Part model, mm, in its own coordinate system. A direction names the side the tool comes from. Give positions to 0.01 mm unless a question says otherwise; leave off trailing zeros. Write each loop counter-clockwise with the first axis right and the second up, starting at its lowest first coordinate (ties: lowest second). Pieces come first, ordered by that corner, then holes. Notation, with made-up numbers: M 20,-8.75 L 62,-8.75 A23 cw 62,20.25 Z; hole C -29.5,64.5 d1. An arc over 180 degrees is marked long. Answer as CSV lines item,"result". Start each with the question number.
1) Tool access for faces 4 (the flat face through (19.648, 8.014, -3.033)), 5 (the flat face through (7, 174, -8)), 6 (the cylindrical face through (12.436, 4.521, -39.309)): list every direction of +Z, -Z, +X, -X, +Y, -Y with a clear straight run to the whole face (end or side of a thin tool).
2) Slice it at A-A, the plane z = -45.59. Give the cut face in (x, y).
3) Slice it at B-B, the plane y = 194.5. Give the cut face in (x, z), plus the area to 4 significant figures.
4) Mould opens along X. For faces 1 (the cylindrical face through (9.74, 8.85, -13.76)), 2 (the flat face through (8, 174, 0)), 3 (the cylindrical face through (16.181, 1.479, -49.215)) say: pulls with the +X half, pulls with the -X half, needs draft (parallel to the pull), parting line crosses it, or undercut.
5) Wall check: line 1 along X through (y, z) = (4.7, -45.59); line 2 along Y through (x, z) = (23, -40); line 3 along Z through (x, y) = (8, 155.5). Give the ranges that are in metal, low to high. Write a range as from..to.
6) Slice it at C-C, the plane y = 117.5. Give the cut face in (x, z), plus the area to 3 significant figures.
7) Pin check, flat tips, straight feed: pin 1 Ø12 at (y, z) = (183, -4.5) entering from -X; pin 2 Ø1.5 at (x, z) = (0, -23.5) entering from +Y; pin 3 Ø8.5 at (x, z) = (15.04, -45.59) entering from +Y. Stop position of each tip, or through.
```python
from build123d import *

# Parameters (mm, degrees)
BOSS_EXTRUDE3_DEPTH = 320
SKETCH7_W           = 15
SKETCH7_H           = 111
CUT_EXTRUDE3_DEPTH  = 321.702354216
BOSS_EXTRUDE5_DEPTH = 140
SKETCH4_R           = 3.8
BOSS_EXTRUDE4_DEPTH = 6
BOSS_EXTRUDE6_DEPTH = 10
CUT_EXTRUDE4_DEPTH  = 220.0148158
SKETCH11_R          = 6.8
CUT_EXTRUDE5_DEPTH  = 3


with BuildPart() as part:
    # Sketch1 → Boss-Extrude3 (new body)
    with BuildSketch(Plane(origin=(0, 0, 0), x_dir=(1, 0, 0), z_dir=(0, 1, 0))):
        Polygon((0, 0), (0, 15), (15, 0), align=None)
    extrude(amount=BOSS_EXTRUDE3_DEPTH)

    # Sketch7 → Cut-Extrude3 (cut, through all)
    with BuildSketch(Plane.XY):
        with Locations((7.5, 264.5)):
            Rectangle(SKETCH7_W, SKETCH7_H)
    extrude(amount=-CUT_EXTRUDE3_DEPTH, mode=Mode.SUBTRACT)

    # Sketch8 → Boss-Extrude5 (add)
    with BuildSketch(Plane.XZ):
        Polygon((-3, -22.242640687), (-3, 3), (22.242640687, 3), align=None)
    extrude(amount=-BOSS_EXTRUDE5_DEPTH)

    # Sketch4 → Boss-Extrude4 (add)
    with BuildSketch(Plane.XZ):
        Polygon((0, -55), (25, -55), (25, 3), (22.242640687, 3), (-3, -22.242640687), (-3, -55), align=None)
        with Locations(Location((15.04, -45.59, 0), (0, 0, 270))):
            Circle(SKETCH4_R, mode=Mode.SUBTRACT)
    extrude(amount=-BOSS_EXTRUDE4_DEPTH)

    # Sketch9 → Boss-Extrude6 (add)
    with BuildSketch(Plane(origin=(0, 6, 0), x_dir=(1, 0, 0), z_dir=(0, 1, 0))):
        Polygon((-3, 22.242640687), (4.071067812, 29.313708499), (25, 8.384776311), (17.928932188, 1.313708499), align=None)
    extrude(amount=BOSS_EXTRUDE6_DEPTH)

    # Sketch10 → Cut-Extrude4 (cut, through all)
    with BuildSketch(Plane(origin=(8.307611845, 0, 8.307611845), x_dir=(0.7071067811865479, 0, -0.7071067811865471), z_dir=(0.7071067811865471, 0, 0.7071067811865479))):
        with BuildLine():
            Line((13.606601718, 16), (23.606601718, 16))
            Line((23.606601718, 16), (23.606601718, 6))
            ThreePointArc((23.606601718, 6), (16.535533906, 8.928932188), (13.606601718, 16))
        make_face()
    extrude(amount=-CUT_EXTRUDE4_DEPTH, mode=Mode.SUBTRACT)

    # Sketch11 → Cut-Extrude5 (cut)
    with BuildSketch(Plane(origin=(0, 6, 0), x_dir=(1, 0, 0), z_dir=(0, 1, 0))):
        with Locations(Location((15.04, 45.59, 0), (0, 0, 270))):
            Circle(SKETCH11_R)
    extrude(amount=-CUT_EXTRUDE5_DEPTH, mode=Mode.SUBTRACT)


solid = part.part
```
Found:
1,face 4,"+X, +Y"
1,face 5,"-Z, +X, +Y"
1,face 6,"+Y"
2,outline,"M -3,0 L 11.24,0 L 11.24,3 L 8.24,3 L 8.24,6 L -3,6 Z; M 18.84,0 L 25,0 L 25,6 L 21.84,6 L 21.84,3 L 18.84,3 Z"
3,outline,"M 0,-15 L 15,0 L 0,0 Z"
3,area,"112.5 mm²"
4,face 1,"pulls with the +X half"
4,face 2,"needs draft"
4,face 3,"undercut"
5,line 1,"-3..8.24, 21.84..25"
5,line 2,"0..6"
5,line 3,"-7..0"
6,outline,"M -3,-22.24 L 22.24,3 L -3,3 Z"
6,area,"319 mm²"
7,pin 1,"x = 0"
7,pin 2,"y = 9.67"
7,pin 3,"y = 3"
